Answer from the drawing. Dimensions are ordinates in mm from the lowest x, y and z of the part. Coordinates: 2 decimals unless noted, no trailing zeros. Write each loop counter-clockwise with the first axis right and the second up, starting at its lowest first coordinate (ties: lowest second). Pieces come first, ordered by that corner, then holes.
(1) Given pin 1 (10 mm diameter, centred on x = 486.5, z = 230.5, fed in from +Y); pin 2 (1 mm diameter, centred on x = 1515, z = 180, fed in from -Y); pin 3 (4 mm diameter, centred on y = 368.5, z = 181, fed in from +X), each flat-ended and moving along its own axis, determine where each tip first touches the part or whether it passes through.
(2) Section D-D on z = 249 is taken. Write down the section's boundary in (x, y).
(3) Find the intervals of material crossed by probe 1 along X at (y, z) = (196, 471); probe 2 along Y at (x, z) = (1399, 463); probe 3 along Z at (x, y) = (264, 180.5), in increasing order.
(4) Section C-C on x = 371 is taken. Write down the section's boundary in (y, z).
(5) Section A-A on y = 355.6 is taken. Write down the section's boundary in (x, z).
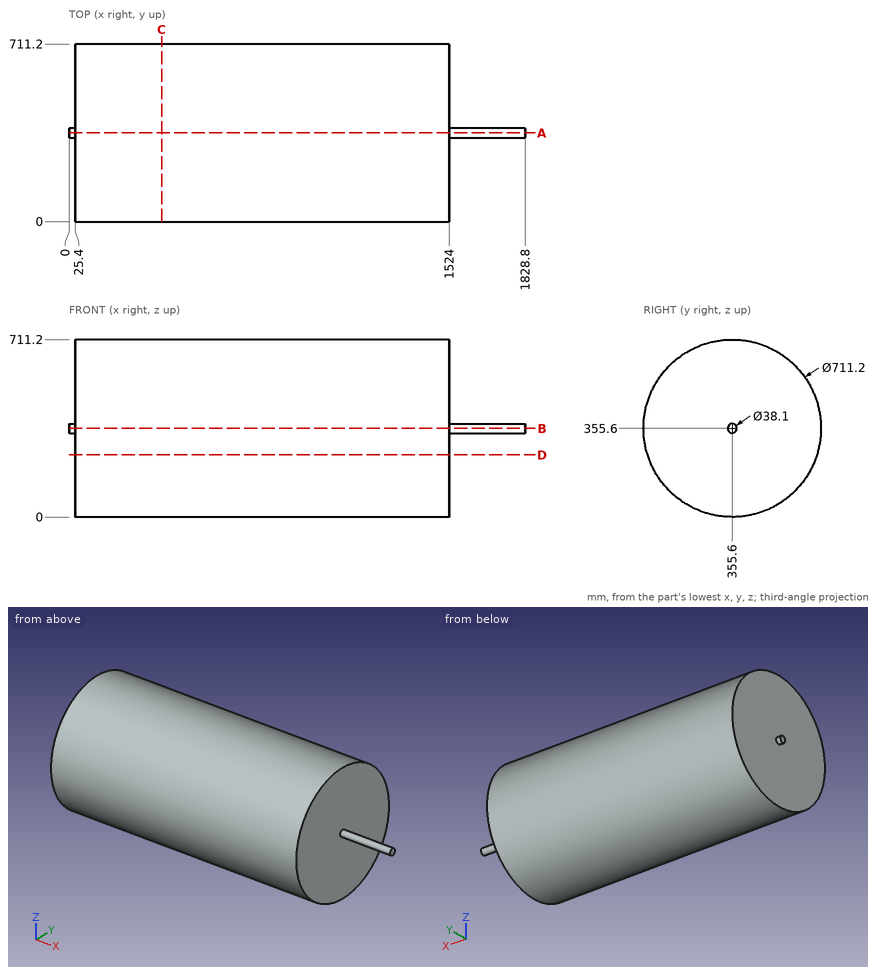
Response:
1. pin 1: stops at y = 690.3
1. pin 2: stops at y = 46.1
1. pin 3: stops at x = 1524
2. outline: (25.4, 16.35) - (1524, 16.35) - (1524, 694.85) - (25.4, 694.85) - close
3. probe 1: x = 25.4 to 1524
3. probe 2: y = 16.61 to 694.59
3. probe 3: z = 46.1 to 665.1
4. outline: circle Ø711.2 at (355.6, 355.6)
5. outline: (0, 336.55) - (25.4, 336.55) - (25.4, 0) - (1524, 0) - (1524, 336.55) - (1828.8, 336.55) - (1828.8, 374.65) - (1524, 374.65) - (1524, 711.2) - (25.4, 711.2) - (25.4, 374.65) - (0, 374.65) - close
